from build123d import *

# Parameters (mm, degrees)
BOSS_EXTRUDE1_DEPTH                 = 5
F_8_CLEARANCE_HOLE1_D               = 4.4958
F_8_CLEARANCE_HOLE1_DEPTH           = 17
F_8_CLEARANCE_HOLE1_TIP             = 1.350674586
SKETCH3_W                           = 6
SKETCH3_H                           = 6
BOSS_EXTRUDE2_DEPTH                 = 15
F_8_CLEARANCE_HOLE2_D               = 4.4958
F_8_CLEARANCE_HOLE2_DEPTH           = 17
F_8_CLEARANCE_HOLE2_TIP             = 1.350674586
F_8_CLEARANCE_HOLE2_ON_FACE_2_D     = 4.4958
F_8_CLEARANCE_HOLE2_ON_FACE_2_DEPTH = 17
F_8_CLEARANCE_HOLE2_ON_FACE_2_TIP   = 1.350674586


with BuildPart() as part:
    # Sketch1 → Boss-Extrude1 (new body)
    with BuildSketch(Plane(origin=(0, 0, 0), x_dir=(1, 0, 0), z_dir=(0, 1, 0))):
        Polygon((-14.338976611, 0), (30.661023389, 0), (30.661023389, 55.621488653), (8.161023389, 55.621488653), (-14.338976611, 55.621488653), align=None)
    extrude(amount=BOSS_EXTRUDE1_DEPTH)

    # #8 Clearance Hole1
    with Locations(Plane(origin=(22.377803879, 0, -10), x_dir=(0, 0, -1), z_dir=(0, -1, 0))):
        with Locations((0, 0), (0, -27.25), (30.001031232, -13.625)):
            Hole(F_8_CLEARANCE_HOLE1_D / 2, depth=F_8_CLEARANCE_HOLE1_DEPTH)
            with Locations((0, 0, -(F_8_CLEARANCE_HOLE1_DEPTH + F_8_CLEARANCE_HOLE1_TIP / 2))):  # 118° drill point
                Cone(0, F_8_CLEARANCE_HOLE1_D / 2, F_8_CLEARANCE_HOLE1_TIP, mode=Mode.SUBTRACT)

    # Sketch3 → Boss-Extrude2 (add)
    with BuildSketch(Plane(origin=(0, 0, 0), x_dir=(-1, 0, 0), z_dir=(0, -1, 0))):
        with Locations((-1.161023389, 47.5)):
            Rectangle(SKETCH3_W, SKETCH3_H)
        with Locations((-1.161023389, 13)):
            Rectangle(SKETCH3_W, SKETCH3_H)
        with Locations((-15.161023389, 47.684631069)):
            Rectangle(SKETCH3_W, SKETCH3_H)
        with Locations((-15.161023389, 12.990172473)):
            Rectangle(SKETCH3_W, SKETCH3_H)
    extrude(amount=BOSS_EXTRUDE2_DEPTH)

    # #8 Clearance Hole2
    with Locations(Plane(origin=(-1.838976611, -11, -47.5), x_dir=(0, 0, -1), z_dir=(-1, 0, 0))):
        with Locations((0, 0), (-34.5, 0)):
            Hole(F_8_CLEARANCE_HOLE2_D / 2, depth=F_8_CLEARANCE_HOLE2_DEPTH)
            with Locations((0, 0, -(F_8_CLEARANCE_HOLE2_DEPTH + F_8_CLEARANCE_HOLE2_TIP / 2))):  # 118° drill point
                Cone(0, F_8_CLEARANCE_HOLE2_D / 2, F_8_CLEARANCE_HOLE2_TIP, mode=Mode.SUBTRACT)

    # #8 Clearance Hole2 on face 2
    with Locations(Plane(origin=(18.161023389, -11, -47.684631069), x_dir=(0, 0, 1), z_dir=(1, 0, 0))):
        with Locations((0, 0), (34.694458596, 0)):
            Hole(F_8_CLEARANCE_HOLE2_ON_FACE_2_D / 2, depth=F_8_CLEARANCE_HOLE2_ON_FACE_2_DEPTH)
            with Locations((0, 0, -(F_8_CLEARANCE_HOLE2_ON_FACE_2_DEPTH + F_8_CLEARANCE_HOLE2_ON_FACE_2_TIP / 2))):  # 118° drill point
                Cone(0, F_8_CLEARANCE_HOLE2_ON_FACE_2_D / 2, F_8_CLEARANCE_HOLE2_ON_FACE_2_TIP, mode=Mode.SUBTRACT)


solid = part.part
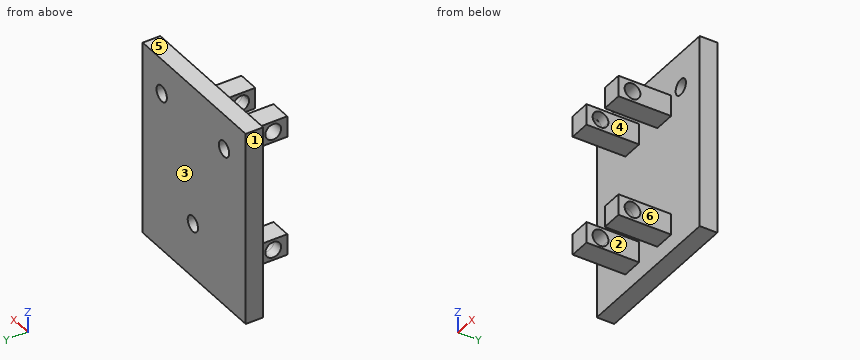
Read the model definition and answer for the solid it produces. Units are mm, in the model's axes. Face numbers are marked on the shaded views. A direction names the side the tool comes from. Round coordinates to 2 decimals unless told otherwise and drop trailing zeros. Loops run counter-clockwise (first coordinate to the right, second up) from the corner with the lowest first, then second, coordinate; pieces in that order, holes last.
Q1. Which of the six approach directions +Z, -Z, +X, -X, +Y, -Y give full straight-line access (tool end or side, diameter ignored) to the marked faces 4, 5 and 6?
Q2. Section B-B on z = -37 is taken. Write down the section's boundary in (x, y).
Q3. Each of these flat-tipped pins is pushed along its axis until it touches: pin 1 (3 mm diameter, centred on x = 14.5, y = -7.5, fed in from -Z); pin 2 (3 mm diameter, centred on y = -8, z = -47.5, fed in from -X); pin 3 (1.8 mm diameter, centred on x = 0.5, y = -8.5, fed in from +Z). Where does it stop, or does it pass through?
Q4. Section C-C on y = -11 is taken. Give the number of separate pieces and of enclosed holes in the cut face, and give its area (3 significant figures).
Q5. Consider probe 1 along X at (y, z) = (1.75, -10); probe 2 along X at (y, z) = (-3, -14); probe 3 along Z at (x, y) = (2.5, -13.5). Determine where each line is inside the solid, lowest interval first.
Q6. Section A-A on y = -6.25 is taken. Write down the section's boundary in (x, z), and give its area (3 significant figures).
Q7. Determine the mould class of the marked faces 1, 2 and 3 for opening direction X: released by +X, released by -X, zero draft, split by the parting line, or undercut.
Output:
1. face 4: +Z, -Z, -Y
1. face 5: +Z, +X, -X, +Y, -Y
1. face 6: +Z, -Z, +X, -Y
2. outline: (-14.34, 0) - (30.66, 0) - (30.66, 5) - (-14.34, 5) - close
3. pin 1: stops at z = -50.68
3. pin 2: stops at x = -1.84
3. pin 3: stops at z = -10
4. separate pieces: 8
4. enclosed holes: 0
4. area: 34.9 mm2
5. probe 1: x = -14.34 to -7.12, -2.62 to 20.13, 24.63 to 30.66
5. probe 2: x = -1.84 to 4.16, 12.16 to 18.16
5. probe 3: z = -50.5 to -44.5, -16 to -10
6. outline: (-1.84, -50.5) - (4.16, -50.5) - (4.16, -44.5) - (-1.84, -44.5) - close; (-1.84, -16) - (4.16, -16) - (4.16, -10) - (-1.84, -10) - close; (12.16, -50.68) - (18.16, -50.68) - (18.16, -44.68) - (12.16, -44.68) - close; (12.16, -15.99) - (18.16, -15.99) - (18.16, -9.99) - (12.16, -9.99) - close
6. area: 144 mm2
7. face 1: released by -X
7. face 2: undercut
7. face 3: zero draft
